```python
from build123d import *

# Parameters (mm, degrees)
SKETCH1_W       = 381
SKETCH1_H       = 63.5
OUTER_CUT_DEPTH = 1.5875
SLOTS_DEPTH     = 194.153806913


with BuildPart() as part:
    # Sketch1 → Outer Cut (new, symmetric)
    with BuildSketch(Plane(origin=(0, 0, 0), x_dir=(0, 0, -1), z_dir=(1, 0, 0))):
        Rectangle(SKETCH1_W, SKETCH1_H)
    extrude(amount=OUTER_CUT_DEPTH, both=True)

    # Sketch2 → Slots (cut, through all)
    with BuildSketch(Plane(origin=(1.5875, 0, 0), x_dir=(0, 0, -1), z_dir=(1, 0, 0))):
        with BuildLine():
            Line((-177.8, 15.875), (177.8, 15.875))
            ThreePointArc((177.8, 15.875), (180.975, 12.7), (177.8, 9.525))
            Line((177.8, 9.525), (-177.8, 9.525))
            ThreePointArc((-177.8, 9.525), (-180.975, 12.7), (-177.8, 15.875))
        make_face()
        with BuildLine():
            Line((-177.8, -15.875), (177.8, -15.875))
            ThreePointArc((177.8, -15.875), (180.975, -12.7), (177.8, -9.525))
            Line((177.8, -9.525), (-177.8, -9.525))
            ThreePointArc((-177.8, -9.525), (-180.975, -12.7), (-177.8, -15.875))
        make_face()
    extrude(amount=-SLOTS_DEPTH, mode=Mode.SUBTRACT)


solid = part.part
```
Source: CAD feature listing. Evaluate the final solid. Frame: model axes, mm. Coordinates: 2 decimals unless noted, no trailing zeros. Loops run counter-clockwise (first coordinate to the right, second up) from the corner with the lowest first, then second, coordinate; pieces in that order, holes last. Notation, with made-up numbers: (37.5, -29.5) -> (56.5, -29.5) arc R19 cw to (56.5, -10.5) -> close; hole circle Ø7 at (60.5, 0). An arc over 180 degrees is marked (long way). One line per item, written item: value. Start each with the question number.
Q1. Section query B-B, the plane z = 101. Give the number of separate pieces and of enclosed holes in the cut face, and give its area (3 significant figures).
Q2. Section query A-A, the plane y = -12.7. Return the cut outline in (x, z) (1 decimal), and give its area (3 significant figures).
Q3. Section query C-C, the plane x = -0.15. Return the cut outline in (y, z) (3 decimals), and give its area (3 significant figures).
Q4. Line query: line 1 along Y through (x, z) = (-0.45, 101.5) (3 decimals); line 2 along Z through (x, y) = (0.75, 14). Output: solid intervals per line, ascending.
Results:
1. separate pieces: 3
1. enclosed holes: 0
1. area: 161 mm^2
2. outline: (-1.6, -190.5) -> (1.6, -190.5) -> (1.6, -181) -> (-1.6, -181) -> close; (-1.6, 181) -> (1.6, 181) -> (1.6, 190.5) -> (-1.6, 190.5) -> close
2. area: 60.5 mm^2
3. outline: (-31.75, -190.5) -> (31.75, -190.5) -> (31.75, 190.5) -> (-31.75, 190.5) -> close; hole (-15.875, -177.8) arc R3.175 ccw to (-9.525, -177.8) -> (-9.525, 177.8) arc R3.175 ccw to (-15.875, 177.8) -> close; hole (9.525, -177.8) arc R3.175 ccw to (15.875, -177.8) -> (15.875, 177.8) arc R3.175 ccw to (9.525, 177.8) -> close
3. area: 19,600 mm^2
4. line 1: -31.75 to -15.875, -9.525 to 9.525, 15.875 to 31.75
4. line 2: -190.5 to -180.7, 180.7 to 190.5
